Part model, mm, in its own coordinate system. A direction names the side the tool comes from. Give positions to 0.01 mm unless a question says otherwise; leave off trailing zeros. Order: outer loops, then holes, each group sorted by start corner. A loop starts at its lowest first (then second) coordinate and runs counter-clockwise, first axis right, second up. Notation, with made-up numbers: M 51,32.5 L 69,32.5 A26 ccw 69,54.5 Z; hole C 61.25,82 d11. An arc over 180 degrees is marked long. Answer as a JSON object with one key per item and string values.
from build123d import *

# Parameters (mm, degrees)
SKETCH_1_W          = 17.5
SKETCH_1_H          = 85
EXTRUDE_1_DEPTH     = 44
SKETCH_2_W          = 17.5
SKETCH_2_H          = 45
EXTRUDE_2_DEPTH     = 15
EXTRUDE_3_DEPTH     = 5
CHAMFER_1_SIZE2     = 3.526539614
CHAMFER_1_SIZE      = 20
CHAMFER_2_SIZE2     = 3.526539614
CHAMFER_2_SIZE      = 20
CHAMFER_3_SIZE      = 2
CHAMFER_3_SIZE_2    = 22.860104606
CHAMFER_4_SIZE      = 2
CHAMFER_4_SIZE_2    = 22.860104606
FILLET_START        = -1
FILLET_1_DEPTH      = 19
FILLET_2_R          = 4
EXTRUDE_5_DEPTH     = 17.5
CUT_EXTRUDE_1_REACH = 110.872
SKETCH_6_W          = 35
SKETCH_6_H          = 4


with BuildPart() as part:
    # Эскиз1 → Бобышка-Вытянуть1 (new body)
    with BuildSketch(Plane(origin=(0, 0, 0), x_dir=(1, 0, 0), z_dir=(0, 1, 0))):
        with Locations((8.75, 42.5)):
            Rectangle(SKETCH_1_W, SKETCH_1_H)
    extrude(amount=EXTRUDE_1_DEPTH)

    # Эскиз2 → Бобышка-Вытянуть2 (add)
    with BuildSketch(Plane(origin=(0, 44, 0), x_dir=(1, 0, 0), z_dir=(0, 1, 0))):
        with Locations((8.75, 42.5)):
            Rectangle(SKETCH_2_W, SKETCH_2_H)
    extrude(amount=EXTRUDE_2_DEPTH)

    # Эскиз3 → Бобышка-Вытянуть3 (add)
    with BuildSketch(Plane(origin=(0, 59, 0), x_dir=(1, 0, 0), z_dir=(0, 1, 0))):
        Polygon((17.5, 42.5), (17.5, 47.5), (0, 47.5), (0, 42.5), (0, 37.5), (17.5, 37.5), align=None)
    extrude(amount=EXTRUDE_3_DEPTH)

    # Фаска1
    chamfer_1_edges = [part.edges().sort_by_distance(p)[0] for p in [
        (8.75, 44, -65),
    ]]
    chamfer_1_side = [part.faces().sort_by_distance(p)[0] for p in [
        (8.75, 44, -65.070530792),
    ]]
    chamfer(chamfer_1_edges, length=CHAMFER_1_SIZE - 0.0001, length2=CHAMFER_1_SIZE2 - 0.0001, reference=chamfer_1_side[0])  # a hair under: the kernel refuses the full size

    # Фаска2
    chamfer_2_edges = [part.edges().sort_by_distance(p)[0] for p in [
        (8.75, 44, -20),
    ]]
    chamfer_2_side = [part.faces().sort_by_distance(p)[0] for p in [
        (8.75, 44, -19.929469208),
    ]]
    chamfer(chamfer_2_edges, length=CHAMFER_2_SIZE - 0.0001, length2=CHAMFER_2_SIZE2 - 0.0001, reference=chamfer_2_side[0])  # a hair under: the kernel refuses the full size

    # Фаска3
    # the kernel refuses this chamfer: 22.860104606, 2 mm, written as the material it takes off along each edge
    with BuildSketch(Plane(origin=(-59.427907001, 59, -65), x_dir=(0, -1, 0), z_dir=(1, 0, 0))) as chamfer_3_piece_1_section:
        Polygon((CHAMFER_3_SIZE, 0), (0, -CHAMFER_3_SIZE_2), (0, 0), align=None)
    chamfer_3_piece_1 = extrude(amount=136.355814002, mode=Mode.PRIVATE)
    chamfer_3_piece_1 = split(chamfer_3_piece_1, bisect_by=Plane(origin=(-59.427907001, 59, -47.5), z_dir=(0, 0, -1)), keep=Keep.TOP, mode=Mode.PRIVATE)
    add(chamfer_3_piece_1, mode=Mode.SUBTRACT)

    # Фаска4
    # the kernel refuses this chamfer: 22.860104606, 2 mm, written as the material it takes off along each edge
    with BuildSketch(Plane(origin=(76.927907001, 59, -20), x_dir=(0, -1, 0), z_dir=(-1, 0, 0))) as chamfer_4_piece_1_section:
        Polygon((CHAMFER_4_SIZE, 0), (0, -CHAMFER_4_SIZE_2), (0, 0), align=None)
    chamfer_4_piece_1 = extrude(amount=136.355814002, mode=Mode.PRIVATE)
    chamfer_4_piece_1 = split(chamfer_4_piece_1, bisect_by=Plane(origin=(76.927907001, 59, -37.5), z_dir=(0, 0, 1)), keep=Keep.TOP, mode=Mode.PRIVATE)
    add(chamfer_4_piece_1, mode=Mode.SUBTRACT)

    # Скругление1: read off the stored shape, not the designer's step
    # Скругление1 outline → Скругление1 (cut)
    with BuildSketch(Plane.YZ.offset(FILLET_START)):
        with BuildLine():
            Line((44, 0), (41.482701106, 0))
            ThreePointArc((41.482701106, 0), (43.411063935, -0.701866671), (44.437124366, -2.479055467))
            Line((44.437124366, -2.479055467), (44, 0))
        make_face()
        with BuildLine():
            Line((57, -20), (54.251006478, -20))
            ThreePointArc((54.251006478, -20), (56.277777101, -20.78816799), (57.239590572, -22.738532772))
            Line((57.239590572, -22.738532772), (57, -20))
        make_face()
        with BuildLine():
            Line((57, -65), (57.239590572, -62.261467228))
            ThreePointArc((57.239590572, -62.261467228), (56.277777101, -64.21183201), (54.251006478, -65))
            Line((54.251006478, -65), (57, -65))
        make_face()
        with BuildLine():
            Line((44, -85), (44.437124366, -82.520944533))
            ThreePointArc((44.437124366, -82.520944533), (43.411063935, -84.298133329), (41.482701106, -85))
            Line((41.482701106, -85), (44, -85))
        make_face()
    extrude(amount=FILLET_1_DEPTH, mode=Mode.SUBTRACT)

    # Скругление2
    fillet_2_edges = [part.edges().sort_by_distance(p)[0] for p in [
        (8.75, 64, -47.5),
        (8.75, 64, -37.5),
    ]]
    fillet(fillet_2_edges, radius=FILLET_2_R)

    # Эскиз5 → Бобышка-Вытянуть5 (add)
    with BuildSketch(Plane.ZY):
        Polygon((-37.808562445, 61.540548206), (-31.915262461, 64), (-32.641917341, 65.741199076), (-39.550806856, 62.857911145), (-38.824151977, 61.11671207), align=None)
    extrude(amount=-EXTRUDE_5_DEPTH)

    # Эскиз6 → Вырез-Вытянуть1 (cut, up to next)
    with BuildSketch(Plane(origin=(17.5, 0, 0), x_dir=(0, 0, -1), z_dir=(1, 0, 0)), mode=Mode.PRIVATE) as cut_extrude_1_sk1:
        with Locations((42.5, 2)):
            Rectangle(SKETCH_6_W, SKETCH_6_H)
    cut_extrude_1_tool1 = extrude(cut_extrude_1_sk1.sketch, amount=-CUT_EXTRUDE_1_REACH, mode=Mode.PRIVATE) & part.part
    add(cut_extrude_1_tool1.solids().sort_by_distance((17.5, 2, -42.5))[0], mode=Mode.SUBTRACT)


solid = part.part
1. Pin check, flat tips, straight feed: P1, Ø2, axis at x = 5.5, z = -38, coming from the +Y side; P2, Ø3, axis at x = 3, y = 58.5, coming from the +Z side; P3, Ø9, axis at x = 5.5, z = -37, coming from the -Y side. Stop position of each tip, or through.
Worked answers:
{"P1": "stops at y = 63.92", "P2": "stops at z = -21.8", "P3": "stops at y = 4"}
2. Cut at A-A on x = 4. Give the cut face in (y, z), plus the area to 3 significant figures.
Worked answers:
{"outline": "M 0,-85 L 41.48,-85 A3 ccw 44.43,-82.53 L 47.53,-65 L 54.25,-65 A3 ccw 57.24,-62.26 L 58.53,-47.5 L 60,-47.5 A4 ccw 64,-43.5 L 64,-41.5 A4 ccw 63.1,-38.97 L 65.74,-32.64 L 64,-31.92 L 61.54,-37.81 A4 ccw 60,-37.5 L 58.53,-37.5 L 57.24,-22.74 A3 ccw 54.25,-20 L 47.53,-20 L 44.43,-2.47 A3 ccw 41.48,0 L 0,0 L 0,-25 L 4,-25 L 4,-60 L 0,-60 Z", "area": "4,350 mm^2"}
3. Two-plate mould, pull along Z, no slides. Class faces 1 (the cylindrical face through (8.872, 63.775, -40.176)), 2 (the cylindrical face through (8.628, 43.384, -0.679)), 3 (the flat face through (17.5, 26, -43)), 4 (the flat face through (8.63, 64.44, -35.76)): +Z half, -Z half, draft (parallel to the pull), parting line (faces both ways), or undercut.
Worked answers:
{"face 1": "undercut", "face 2": "+Z half", "face 3": "draft", "face 4": "undercut"}
4. Cut at C-C on y = 56. Give the cut face in (x, z).
Worked answers:
{"outline": "M 0,-64.44 L 17.5,-64.44 L 17.5,-20.56 L 0,-20.56 Z"}
5. Probe line 1 along Y through (x, z) = (8.25, -35); line 2 along Y through (x, z) = (11.25, -76.5); line 3 along Z through (x, y) = (5.5, 50). List the from-to ranges inside material, lowest first.
Worked answers:
{"line 1": "y = 4 to 58.31, 62.71 to 64.76", "line 2": "y = 0 to 45.5", "line 3": "z = -65 to -20"}
6. Cut at B-B on z = -18. Give the cut face in (x, y), plus the area to 3 significant figures.
Worked answers:
{"outline": "M 0,0 L 17.5,0 L 17.5,47.17 L 0,47.17 Z", "area": "826 mm^2"}
7. Which spindle directions (+Z, -Z, +X, -X, +Y, -Y) get a long thin tool onto all of the face, cutting with end or side? Do faces 5 (the flat face through (8.873, 57.876, -30.016)), 6 (the flat face through (8.628, 46.002, -11.356)), 7 (the flat face through (9, 4, -42)), 8 (the flat face through (9, 64, -43)). Say none if no direction does.
Worked answers:
{"face 5": "+Z, +X, -X", "face 6": "+Z, +X, -X, +Y", "face 7": "+X, -X, -Y", "face 8": "-Z, +X, -X, +Y"}
